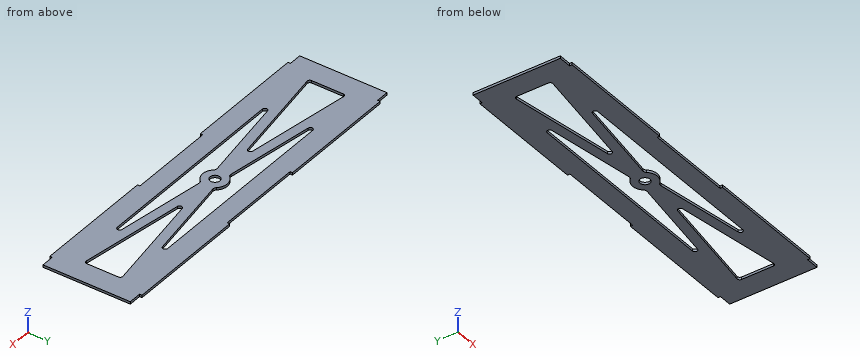
```python
from build123d import *

# Parameters (mm, degrees)
SKETCH_1_W               = 290
SKETCH_1_H               = 71
EXTRUDE_1_DEPTH          = 2
SKETCH_2_W               = 99
SKETCH_2_H               = 4
EXTRUDE_2_DEPTH          = 2
MIRROR_2_COPY_1_SKETCH_W = 99
MIRROR_2_COPY_1_SKETCH_H = 4
MIRROR_2_COPY_1_DEPTH    = 2
CUT_EXTRUDE_1_DEPTH      = 2
SKETCH_4_R               = 10
EXTRUDE_3_DEPTH          = 2
SKETCH_5_R               = 4
CUT_EXTRUDE_2_DEPTH      = 119
FILLET_1_R               = 2
FILLET_2_R               = 3


with BuildPart() as part:
    # 草图1 → 凸台-拉伸1 (new body)
    with BuildSketch(Plane.XY):
        Rectangle(SKETCH_1_W, SKETCH_1_H)
    extrude(amount=EXTRUDE_1_DEPTH)

    # 草图2 → 凸台-拉伸2 (add)
    with BuildSketch(Plane.XY.offset(2)):
        with Locations((-85, 35.5)):
            Rectangle(SKETCH_2_W, SKETCH_2_H)
    extrude_2 = extrude(amount=-EXTRUDE_2_DEPTH)

    # 镜向1: 凸台-拉伸2 across plane
    add(extrude_2.mirror(Plane(origin=(0, 0, 0), x_dir=(0, 0, 1), z_dir=(1, 0, 0))))

    # 镜向2: 凸台-拉伸2 across plane
    add(extrude_2.mirror(Plane.ZX))

    # 镜向2 copy 1 sketch → 镜向2 copy 1 (add)
    with BuildSketch(Plane(origin=(0, 0, 2), x_dir=(-1, 0, 0), z_dir=(0, 0, 1))):
        with Locations((-85, 35.5)):
            Rectangle(MIRROR_2_COPY_1_SKETCH_W, MIRROR_2_COPY_1_SKETCH_H)
    extrude(amount=-MIRROR_2_COPY_1_DEPTH)

    # 草图3 → 切除-拉伸1 (cut)
    with BuildSketch(Plane.XY.offset(2)):
        with BuildLine():
            Line((-122, -20.5), (122, -20.5))
            ThreePointArc((122, -20.5), (125.535533906, -19.035533906), (127, -15.5))
            Line((127, -15.5), (127, 15.5))
            ThreePointArc((127, 15.5), (125.535533906, 19.035533906), (122, 20.5))
            Line((122, 20.5), (-122, 20.5))
            ThreePointArc((-122, 20.5), (-125.535533906, 19.035533906), (-127, 15.5))
            Line((-127, 15.5), (-127, -15.5))
            ThreePointArc((-127, -15.5), (-125.535533906, -19.035533906), (-122, -20.5))
        make_face()
    extrude(amount=-CUT_EXTRUDE_1_DEPTH, mode=Mode.SUBTRACT)

    # 草图4 → 凸台-拉伸3 (add)
    # profile 1 of 4: a face of its own
    with BuildSketch(Plane.XY.offset(2)):
        Polygon((-145, 35.5), (-145, -35.5), (-134.5, -35.5), (-134.5, -37.5), (-35.5, -37.5), (-35.5, -35.5), (35.5, -35.5), (35.5, -37.5), (134.5, -37.5), (134.5, -35.5), (145, -35.5), (145, 35.5), (134.5, 35.5), (134.5, 37.5), (35.5, 37.5), (35.5, 35.5), (-35.5, 35.5), (-35.5, 37.5), (-134.5, 37.5), (-134.5, 35.5), align=None)
        Polygon((-127, 15.2118729), (-130.048778092, 15.67417323), (-124.935850494, 22.990325911), (-108.512649841, 20.5), (108.512649841, 20.5), (124.935850494, 22.990325911), (132.904602809, 16.107215147), (127, 15.2118729), (127, -15.2118729), (132.970266959, -16.117172106), (124.935850494, -22.990325911), (108.512649841, -20.5), (-108.512649841, -20.5), (-124.935850494, -22.990325911), (-130.138762831, -15.687818033), (-127, -15.2118729), align=None, mode=Mode.SUBTRACT)
    # profile 2 of 4: a face of its own
    with BuildSketch(Plane.XY.offset(2)):
        Circle(SKETCH_4_R)
    # profile 3 of 4: a face of its own
    with BuildSketch(Plane.XY.offset(2)):
        with BuildLine():
            Line((122, 20.5), (108.512649841, 20.5))
            Line((108.512649841, 20.5), (8.461883449, 5.32883932))
            ThreePointArc((8.461883449, 5.32883932), (9.607778996, 2.773189996), (10, 0))
            ThreePointArc((10, 0), (9.607778996, -2.773189996), (8.461883449, -5.32883932))
            Line((8.461883449, -5.32883932), (108.512649841, -20.5))
            Line((108.512649841, -20.5), (122, -20.5))
            ThreePointArc((122, -20.5), (125.535533906, -19.035533906), (127, -15.5))
            Line((127, -15.5), (127, -15.2118729))
            Line((127, -15.2118729), (26.68074467, 0))
            Line((26.68074467, 0), (127, 15.2118729))
            Line((127, 15.2118729), (127, 15.5))
            ThreePointArc((127, 15.5), (125.535533906, 19.035533906), (122, 20.5))
        make_face()
    # profile 4 of 4: a face of its own
    with BuildSketch(Plane.XY.offset(2)):
        with BuildLine():
            Line((-127, 15.5), (-127, 15.2118729))
            Line((-127, 15.2118729), (-26.68074467, 0))
            Line((-26.68074467, 0), (-127, -15.2118729))
            Line((-127, -15.2118729), (-127, -15.5))
            ThreePointArc((-127, -15.5), (-125.535533906, -19.035533906), (-122, -20.5))
            Line((-122, -20.5), (-108.512649841, -20.5))
            Line((-108.512649841, -20.5), (-8.461883449, -5.32883932))
            ThreePointArc((-8.461883449, -5.32883932), (-10, 0), (-8.461883449, 5.32883932))
            Line((-8.461883449, 5.32883932), (-108.512649841, 20.5))
            Line((-108.512649841, 20.5), (-122, 20.5))
            ThreePointArc((-122, 20.5), (-125.535533906, 19.035533906), (-127, 15.5))
        make_face()
    extrude(amount=-EXTRUDE_3_DEPTH)

    # 草图5 → 切除-拉伸2 (cut)
    with BuildSketch(Plane.XY.offset(2)):
        Circle(SKETCH_5_R)
    extrude(amount=-CUT_EXTRUDE_2_DEPTH, mode=Mode.SUBTRACT)

    # 圆角1
    fillet_1_edges = [part.edges().sort_by_distance(p)[0] for p in [
        (108.512649841, -20.5, 1),
        (127, -15.2118729, 1),
        (26.68074467, 0, 1),
        (127, 15.2118729, 1),
        (108.512649841, 20.5, 1),
        (-108.512649841, 20.5, 1),
        (-127, 15.2118729, 1),
        (-26.68074467, 0, 1),
        (-127, -15.2118729, 1),
        (-108.512649841, -20.5, 1),
    ]]
    fillet(fillet_1_edges, radius=FILLET_1_R)

    # 圆角2
    fillet_2_edges = [part.edges().sort_by_distance(p)[0] for p in [
        (8.461883449, -5.32883932, 1),
        (8.461883449, 5.32883932, 1),
        (-8.461883449, 5.32883932, 1),
        (-8.461883449, -5.32883932, 1),
    ]]
    fillet(fillet_2_edges, radius=FILLET_2_R)


solid = part.part
```
Here's how the part is built. I have some questions about the finished solid (model axes, mm). Give positions to 0.01 mm unless a question says otherwise; leave off trailing zeros. Order: outer loops, then holes, each group sorted by start corner. A loop starts at its lowest first (then second) coordinate and runs counter-clockwise, first axis right, second up. Notation, with made-up numbers: (4.5, -16.75) - (27.5, -16.75) arc R15 cw to (27.5, -12.75) - close; hole circle Ø1 at (-15, 47). An arc over 180 degrees is marked (long way). Answer as a JSON object with one key per item and string values. Group by question number.
Item 1: If we section it at B-B on z = 1.6: Give the number of separate pieces and of enclosed holes in the cut face, and give its area (3 significant figures).
Item 2: Please list where these lines run through material, in increasing order: probe 1 along Y at (x, z) = (0, 1.25); probe 2 along Y at (x, z) = (-63, 1); probe 3 along Y at (x, z) = (111.5, 1.3).
Item 3: If we section it at A-A on x = 0: Please give me the cut outline in (y, z).
Item 4: If we section it at C-C on x = 55: Please give me the cut outline in (y, z).
Item 5: For P1, Ø1, axis at y = 36.5, z = 1, coming from the +X side; P2, Ø0.6, axis at x = -139.5, z = 1, coming from the -Y side; P3, Ø1, axis at y = 36.5, z = 1.5, coming from the -X side, each with a flat end and sliding along its axis, tell me the tip position at first contact or that it passes through.
Result set:
{
 "1": {"separate pieces": "1", "enclosed holes": "5", "area": "15,100 mm²"},
 "2": {"probe 1": "-35.5 to -20.5, -10 to -4, 4 to 10, 20.5 to 35.5", "probe 2": "-37.5 to -20.5, -13.6 to -5.51, 5.51 to 13.6, 20.5 to 37.5", "probe 3": "-37.5 to -12.86, 12.86 to 37.5"},
 "3": {"outline": "(-35.5, 0) - (-20.5, 0) - (-20.5, 2) - (-35.5, 2) - close; (-10, 0) - (-4, 0) - (-4, 2) - (-10, 2) - close; (4, 0) - (10, 0) - (10, 2) - (4, 2) - close; (20.5, 0) - (35.5, 0) - (35.5, 2) - (20.5, 2) - close"},
 "4": {"outline": "(-37.5, 0) - (-20.5, 0) - (-20.5, 2) - (-37.5, 2) - close; (-12.39, 0) - (-4.29, 0) - (-4.29, 2) - (-12.39, 2) - close; (4.29, 0) - (12.39, 0) - (12.39, 2) - (4.29, 2) - close; (20.5, 0) - (37.5, 0) - (37.5, 2) - (20.5, 2) - close"},
 "5": {"P1": "x = 134.5", "P2": "y = -35.5", "P3": "x = -134.5"}
}
